from build123d import *

# Parameters (mm, degrees)
BOSS_EXTRUDE1_DEPTH = 16
BOSS_EXTRUDE2_DEPTH = 16
BOSS_EXTRUDE3_DEPTH = 42
BOSS_EXTRUDE4_DEPTH = 12


with BuildPart() as part:
    # Sketch1 → Boss-Extrude1 (new body)
    with BuildSketch(Plane(origin=(0, 0, 0), x_dir=(1, 0, 0), z_dir=(0, 1, 0))):
        with BuildLine():
            Line((0, 64), (0, 0))
            Line((0, 0), (96, 0))
            Line((96, 0), (96, 16))
            Line((96, 16), (76, 16))
            ThreePointArc((76, 16), (68, 24), (76, 32))
            Line((76, 32), (96, 32))
            Line((96, 32), (96, 64))
            Line((96, 64), (0, 64))
        make_face()
    extrude(amount=BOSS_EXTRUDE1_DEPTH)

    # Sketch2 → Boss-Extrude2 (add)
    with BuildSketch(Plane.ZY):
        with BuildLine():
            Line((0, 0), (-64, 0))
            Line((-64, 0), (-64, 64))
            Line((-64, 64), (-48, 64))
            ThreePointArc((-48, 64), (-14.058874503, 49.941125497), (0, 16))
            Line((0, 16), (0, 0))
        make_face()
    extrude(amount=-BOSS_EXTRUDE2_DEPTH)

    # Sketch3 → Boss-Extrude3 (add)
    with BuildSketch(Plane(origin=(0, 0, -64), x_dir=(-1, 0, 0), z_dir=(0, 0, -1))):
        with BuildLine():
            Line((-56, 16), (-16, 16))
            Line((-16, 16), (-16, 41))
            Line((-16, 41), (-24, 41))
            ThreePointArc((-24, 41), (-36, 29), (-48, 41))
            Line((-48, 41), (-56, 41))
            Line((-56, 41), (-56, 16))
        make_face()
    extrude(amount=-BOSS_EXTRUDE3_DEPTH)

    # Sketch4 → Boss-Extrude4 (add)
    with BuildSketch(Plane(origin=(0, 0, -64), x_dir=(-1, 0, 0), z_dir=(0, 0, -1))):
        Polygon((-96, 16), (-56, 41), (-56, 16), align=None)
    extrude(amount=-BOSS_EXTRUDE4_DEPTH)


solid = part.part
Design review of the part built by this model. Coordinates are the model's own, in mm. A direction names the side the tool comes from. Round coordinates to 2 decimals unless told otherwise and drop trailing zeros. Write each loop counter-clockwise with the first axis right and the second up, starting at its lowest first coordinate (ties: lowest second). Pieces come first, ordered by that corner, then holes. Notation, with made-up numbers: (35, -4) - (57, -4) arc R23 ccw to (57, 23) - close; hole circle Ø7 at (-12.5, 73.5). An arc over 180 degrees is marked (long way). Return JSON: item names as keys, results as strings. Group by question number.
Item 1: We need section D-D on z = -24. Write out the cut boundary in (x, y), and give its area (3 significant figures).
Item 2: The part is to be moulded in two halves that separate along Z. For faces 1 (the face through (37, 25, -64)), 2 (the face through (20, 41, -43)), 3 (the face through (7.89, 50.31, -14.43)), 4 (the face through (86, 8, -16)), say which applies: pulls with the +Z half, pulls with the -Z half, needs draft (parallel to the pull), parting line crosses it, or undercut.
Item 3: For probe 1 along Y at (x, z) = (20, -16.5); probe 2 along Y at (x, z) = (19, -24), list the stretches that pass through material, from the lowest coordinate up. Write a range as [from, to].
Item 4: Machinability: for faces 5 (the face through (67, 23, -52)), 6 (the face through (52, 41, -43)), 7 (the face through (96, 8, -48)), 8 (the face through (36, 29, -43)), 9 (the face through (86, 8, -32)), which of the approach directions +Z, -Z, +X, -X, +Y, -Y give a long, thin tool a straight path to every point of the face, cutting with its end or side? Answer none if there is none.
Item 5: We need section A-A on x = 72. Write out the cut boundary in (y, z).
Item 6: We need section B-B on z = -58. Write out the cut boundary in (x, y).
Item 7: Insertion check: P1, Ø3, axis at y = 22.5, z = -12, coming from the -X side; P2, Ø2.5, axis at x = 19, z = -51, coming from the +Y side; P3, Ø24, axis at y = 31.5, z = -24, coming from the +X side. Each pin has a flat end and moves straight along its axis. Give the tip position at first contact, or say it passes through.
Item 8: We need section C-C on x = 36. Write out the cut boundary in (y, z), and give its area (3 significant figures).
Model answer:
{
 "1": {"outline": "(0, 0) - (68, 0) - (68, 16) - (56, 16) - (56, 41) - (48, 41) arc R12 cw to (24, 41) - (16, 41) - (16, 57.57) - (0, 57.57) - close", "area": "2,530 mm²"},
 "2": {"face 1": "pulls with the -Z half", "face 2": "needs draft", "face 3": "pulls with the +Z half", "face 4": "undercut"},
 "3": {"probe 1": "y = [0, 16]", "probe 2": "y = [0, 41]"},
 "4": {"face 5": "+Z, +X, +Y", "face 6": "+Z, -Z, +X, +Y", "face 7": "+Z, -Z, +X, +Y, -Y", "face 8": "+Z, -Z, +Y", "face 9": "+X, +Y, -Y"},
 "5": {"outline": "(0, -64) - (31, -64) - (31, -52) - (16, -52) - (16, -30.93) - (0, -30.93) - close; (0, -17.07) - (16, -17.07) - (16, 0) - (0, 0) - close"},
 "6": {"outline": "(0, 0) - (96, 0) - (96, 16) - (56, 41) - (48, 41) arc R12 cw to (24, 41) - (16, 41) - (16, 64) - (0, 64) - close"},
 "7": {"P1": "stops at x = 0", "P2": "stops at y = 41", "P3": "stops at x = 56"},
 "8": {"outline": "(0, -64) - (29, -64) - (29, -22) - (16, -22) - (16, 0) - (0, 0) - close", "area": "1,570 mm²"}
}
